Can you work these out from the model? Positions are in its coordinate system, mm. Face numbers are marked on the shaded views. A direction names the side the tool comes from. Give positions to 0.01 mm unless a question says otherwise; leave off trailing zeros. Write each loop counter-clockwise with the first axis right and the second up, starting at its lowest first coordinate (ties: lowest second). Pieces come first, ordered by that corner, then holes. Notation, with made-up numbers: M 50,-29.75 L 106,-29.75 A13 ccw 106,-6.75 Z; hole C -16,-38 d2. An arc over 180 degrees is marked long. Write each question's results on one line, items separated by ' | '.
Autodesk Inventor part; units mm, degrees
ref_plane "YZ Plane" through (0, 0, 0) normal (1, 0, 0) x (0, 1, 0)
ref_plane "XZ Plane" through (0, 0, 0) normal (0, 1, 0) x (-1, 0, 0)
ref_plane "XY Plane" through (0, 0, 0) normal (0, 0, 1) x (1, 0, 0)
sketch "Sketch1" plane through (0, 0, 0) normal (0, 0, 1) x (1, 0, 0)
  line L0 (0, 0) -> (50.8, 0)
  line L1 (0, 0) -> (0, 63.5)
  line L2 (0, 63.5) -> (3.175, 63.5)
  line L3 (3.175, 63.5) -> (3.175, 3.175)
  line L4 (3.175, 3.175) -> (50.8, 3.175)
  line L5 (50.8, 3.175) -> (50.8, 0)
  dimension "d0" = 50.8
  dimension "d1" = 63.5
  dimension "d2" = 3.175
extrude "Extrusion1" add sketch "Sketch1" along normal blind 44.45
sketch "Sketch2" plane through (0, 0, 0) normal (-1, 0, 0) x (0, 0, 1)
  line L0 (0, 0) -> (44.45, 0)
  line L1 (0, 63.5) -> (44.45, 63.5)
  line L2 (22.225, 63.5) -> (22.225, 0) construction
  line L3 (11.1125, 47.625) -> (33.3375, 47.625) construction
  circle A0 centre (11.1125, 47.625) radius 2.3812
  circle A1 centre (33.3375, 47.625) radius 2.3813
  circle A2 centre (22.225, 22.225) radius 9.525
  line L4 (0, 63.5) -> (0, 0)
  line L5 (44.45, 63.5) -> (44.45, 0)
  line L6 (0, 53.975) -> (44.45, 53.975)
  line L7 (6.35, 38.1) -> (38.1, 38.1) construction
  circle A3 centre (6.35, 38.1) radius 2.3813
  circle A4 centre (38.1, 38.1) radius 2.3813
  point P0 (22.225, 47.625)
  point P1 (22.225, 38.1)
  dimension "d5" = 22.225
  dimension "d6" = 15.875
  dimension "d7" = 4.7625
  dimension "d8" = 4.7625
  dimension "d11" = 19.05
  dimension "d12" = 22.225
  dimension "d30" = 9.525
  dimension "d31" = 15.875
  dimension "d32" = 31.75
extrude "Extrusion2" cut sketch "Sketch2" against normal blind 38.1 contours L4 L1 L5 L6 | A0 | A1 | A2 | A3 | A4
sketch "Sketch3" plane through (0, 0, 0) normal (0, -1, 0) x (1, 0, 0)
  line L0 (50.8, 0) -> (50.8, 44.45)
  line L1 (0, 0) -> (0, 44.45)
  circle A0 centre (10.795, 31.75) radius 2.3813
  line L2 (10.795, 31.75) -> (10.795, 12.7) construction
  circle A1 centre (10.795, 12.7) radius 2.3813
  line L3 (0, 22.225) -> (50.8, 22.225) construction
  line L4 (0, 0) -> (50.8, 0)
  line L5 (0, 44.45) -> (50.8, 44.45)
  line L6 (41.275, 44.45) -> (41.275, 0)
  circle A2 centre (37.465, 31.75) radius 2.3813
  circle A3 centre (37.465, 12.7) radius 2.3813
  point P0 (10.795, 22.225)
  dimension "d13" = 19.05
  dimension "d17" = 4.7625
  dimension "d18" = 10.795
  dimension "d21" = 41.275
  dimension "d24" = 26.67
extrude "Extrusion3" cut sketch "Sketch3" against normal blind 25.4 contours L4 L6 L5 L0 | A0 | A1 | A2 | A3
fillet "Fillet1" radius 3.175 4 edges at (41.275, 1.5875, 44.45) (41.275, 1.5875, 0) (1.5875, 53.975, 44.45) (1.5875, 53.975, 0)
properties part number "Angle Aluminum P60 Mount" material "Aluminum 6061"
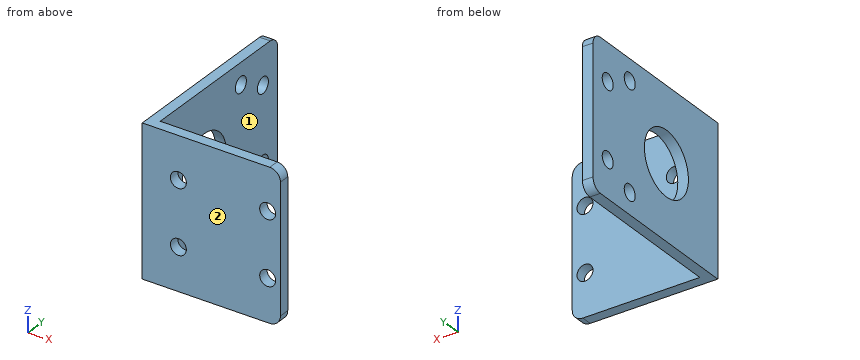
Item 1: I want a section at C-C, the plane y = 24.5. Please give me the cut outline in (x, z) (3 decimals).
Geometry says:
outline: M 0,0 L 3.175,0 L 3.175,12.976 L 0,12.976 Z; M 0,31.474 L 3.175,31.474 L 3.175,44.45 L 0,44.45 Z
Item 2: For the marked faces 1 and 2, which set-ups out of +Z, -Z, +X, -X, +Y, -Y let a thin tool reach every point of the face, with its end or its side?
Geometry says:
face 1: +Z, -Z, +X, +Y | face 2: +Z, -Z, +X, -X, -Y
Item 3: I want a section at A-A, the plane y = 38.1. Please give me the cut outline in (x, z) (3 decimals).
Geometry says:
outline: M 0,0 L 3.175,0 L 3.175,3.969 L 0,3.969 Z; M 0,8.731 L 3.175,8.731 L 3.175,35.719 L 0,35.719 Z; M 0,40.481 L 3.175,40.481 L 3.175,44.45 L 0,44.45 Z
Item 4: I'm going to push flat-ended pins straight in: pin 1 (11.5 mm diameter, centred on x = 15.5, z = 20, fed in from +Y) (3 decimals); pin 2 (17 mm diameter, centred on y = 22.225, z = 22.225, fed in from +X); pin 3 (8 mm diameter, centred on y = 12.5, z = 35.5, fed in from +X) (3 decimals). Where does each tip first touch, or does it pass through?
Geometry says:
pin 1: stops at y = 3.175 | pin 2: passes through | pin 3: stops at x = 3.175
Item 5: If I drill on line 1 (Y direction, x = 31.5, z = 5) (3 decimals), over which ranges is the centre line in solid material (lowest first)? Write a range as from..to.
Geometry says:
line 1: y = 0..3.175
Item 6: I want a section at B-B, the plane z = 6.35. Please give me the cut outline in (x, y) (3 decimals).
Geometry says:
outline: M 0,0 L 41.275,0 L 41.275,3.175 L 3.175,3.175 L 3.175,35.719 L 0,35.719 Z; M 0,40.481 L 3.175,40.481 L 3.175,53.975 L 0,53.975 Z
Item 7: I want a section at D-D, the plane x = 10. Please give me the cut outline in (y, z) (3 decimals), and give its area (3 significant figures).
Geometry says:
outline: M 0,0 L 3.175,0 L 3.175,10.455 L 0,10.455 Z; M 0,14.945 L 3.175,14.945 L 3.175,29.505 L 0,29.505 Z; M 0,33.995 L 3.175,33.995 L 3.175,44.45 L 0,44.45 Z | area: 113 mm2
